Autodesk Inventor part; units mm, degrees
ref_plane "YZ Plane" through (0, 0, 0) normal (1, 0, 0) x (0, 1, 0)
ref_plane "XZ Plane" through (0, 0, 0) normal (0, 1, 0) x (-1, 0, 0)
ref_plane "XY Plane" through (0, 0, 0) normal (0, 0, 1) x (1, 0, 0)
sketch "Sketch1" plane through (0, 0, 0) normal (0, 0, 1) x (1, 0, 0)
  line L0 (0, 6) -> (6, 6)
  line L1 (6, 6) -> (6, 0)
  line L2 (6, 0) -> (0, 0)
  line L3 (0, 0) -> (0, 6)
  dimension "d0" = 6
  dimension "d1" = 6
extrude "Extrusion1" add sketch "Sketch1" along normal blind 300
sketch "Sketch3" plane through (0, 0, 0) normal (0, 1, 0) x (-1, 0, 0)
  line L0 (-6, 300) -> (0, 300) construction
  line L1 (-6, 0) -> (-6, 300) construction
  line L2 (0, 0) -> (0, 300) construction
  line L3 (0, 0) -> (-6, 0) construction
  line L4 (-3, 0) -> (-3, 300) construction
  line L5 (0, 300) -> (-6, 300)
  line L6 (-6, 0) -> (0, 0)
  point P0 (-3, 227)
  point P1 (-3, 98)
  point P2 (-3, 272)
  point P3 (-3, 3)
  dimension "d8" = 129
  dimension "d17" = 73
  dimension "d18" = 28
  dimension "d19" = 3
hole "Hole1" at (3, 0, 227) at (3, 0, 98) at (3, 0, 3) at (3, 0, 272) direction (0, 1, 0) diameter 3 end through all
sketch "Sketch4" plane through (0, 0, 0) normal (-1, 0, 0) x (0, 0, 1)
  line L0 (0, 0) -> (0, 6) construction
  line L1 (0, 0) -> (300, 0) construction
  line L2 (300, 6) -> (300, 0) construction
  line L3 (0, 6) -> (300, 6) construction
  line L4 (0, 0) -> (0, 6) construction
  line L5 (0, 3) -> (300, 3) construction
  line L6 (300, 6) -> (300, 0) construction
  point P0 (266, 3)
  point P1 (9, 3)
  dimension "d20" = 9
  dimension "d21" = 34
hole "Hole2" at (0, 3, 266) at (0, 3, 9) direction (1, 0, 0) diameter 3 end through all
equation "\"d1\" = d0"
properties part number "longitudinal" material "Aluminum"
Read the model definition and answer for the solid it produces. Units are mm, in the model's axes. Round coordinates to 2 decimals unless told otherwise and drop trailing zeros. Order: outer loops, then holes, each group sorted by start corner. A loop starts at its lowest first (then second) coordinate and runs counter-clockwise, first axis right, second up. Notation, with made-up numbers: (-7, 63) - (8, 63) arc R20 ccw to (8, 100) - close; hole circle Ø9 at (64.5, 27). An arc over 180 degrees is marked (long way). Use one line per item in the form item = value. Start each with the question number.
(1) A flat-ended cylindrical pin translates along its axis: pin 1 Ø3.5 at (y, z) = (3, 266) entering from +X. Find the tip coordinate at first contact, or state that the pin passes through.
(2) The part is cut by section A-A (x = 3). Give the vertices of the cut face in (y, z).
(3) Find the intervals of material crossed by line 1 along Z through (x, y) = (3, 1.2); line 2 along X through (y, z) = (4.3, 272), in increasing order. Write a range as from..to.
(4) The part is cut by section B-B (y = 3). Give the vertices of the cut face in (x, z), then the cut area to 3 significant figures.
Checked values:
q1.pin_1 = 6
q2.outline = (0, 0) - (6, 0) - (6, 1.5) - (0, 1.5) - close; (0, 4.5) - (6, 4.5) - (6, 96.5) - (0, 96.5) - close; (0, 99.5) - (6, 99.5) - (6, 225.5) - (0, 225.5) - close; (0, 228.5) - (6, 228.5) - (6, 270.5) - (0, 270.5) - close; (0, 273.5) - (6, 273.5) - (6, 300) - (0, 300) - close; hole circle Ø3 at (3, 9); hole circle Ø3 at (3, 266)
q3.line_1 = 0..1.5, 4.5..96.5, 99.5..225.5, 228.5..270.5, 273.5..300
q3.line_2 = 0..1.5, 4.5..6
q4.outline = (0, 0) - (6, 0) - (6, 7.5) - (0, 7.5) - close; (0, 10.5) - (6, 10.5) - (6, 264.5) - (0, 264.5) - close; (0, 267.5) - (6, 267.5) - (6, 300) - (0, 300) - close; hole circle Ø3 at (3, 3); hole circle Ø3 at (3, 98); hole circle Ø3 at (3, 227); hole circle Ø3 at (3, 272)
q4.area = 1,740 mm^2
